Job drawing, mm, ordinate dimensions from the low corner. One solid piece. Give positions to 0.01 mm unless a question says otherwise; leave off trailing zeros. Order: outer loops, then holes, each group sorted by start corner. A loop starts at its lowest first (then second) coordinate and runs counter-clockwise, first axis right, second up.
Item 1: Band-saw the part on D-D on x = 29. Give the cut face in (y, z).
Item 2: Flat gauge pins, fed straight in: P1, Ø4, axis at x = 25.14, z = 22, coming from the +Y side; P2, Ø2.5, axis at x = 53.5, y = 2.5, coming from the +Z side (1 decimal). Where does each tip first touch, or does it go through?
Item 3: Band-saw the part on C-C on z = 35.5. Give the cut face in (x, y).
Item 4: Band-saw the part on A-A on z = 10.5. Give the cut face in (x, y) (1 decimal).
Item 5: Wall check: L1, parallel to Y at x = 32, z = 16; L2, parallel to Z at x = 30, y = 3; L3, parallel to X at y = 4.5, z = 20.5 (1 decimal). Give the ranges that are in metal, low to high.
Item 6: Band-saw the part on B-B on x = 51. Give the cut face in (y, z).
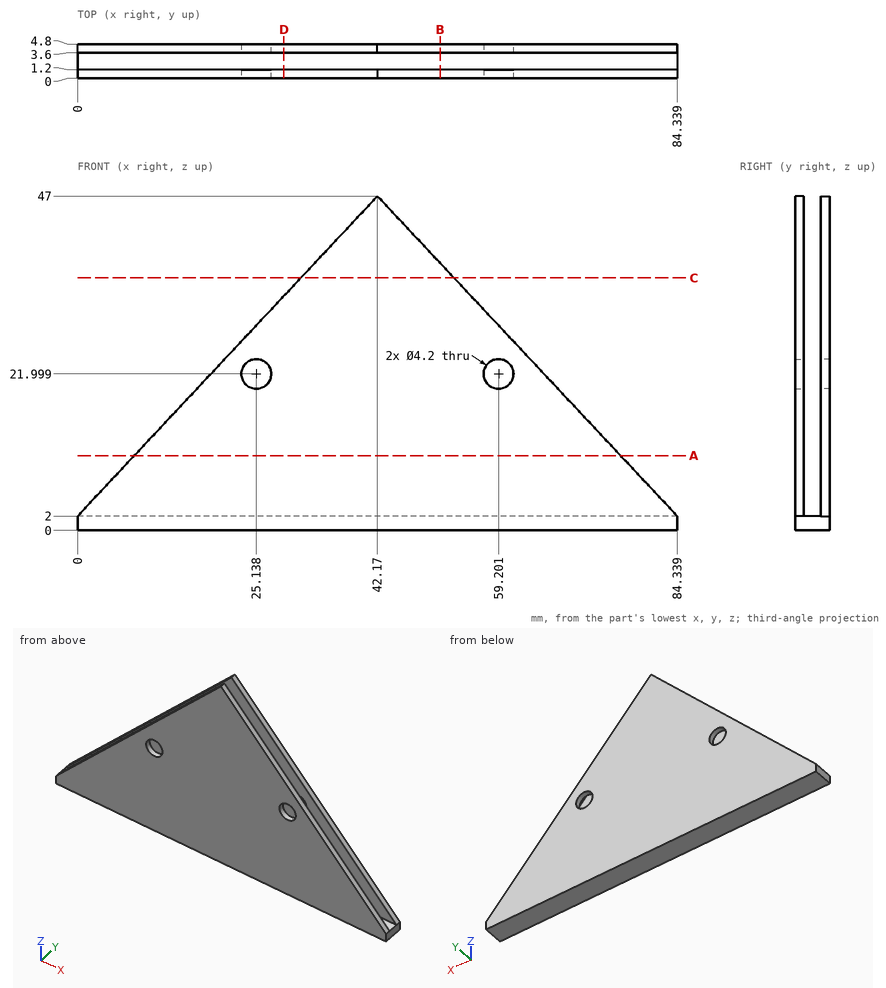
The answers:
1. outline: (0, 0) - (4.8, 0) - (4.8, 32.95) - (3.6, 32.95) - (3.6, 2) - (1.2, 2) - (1.2, 32.95) - (0, 32.95) - close
2. P1: passes through
2. P2: stops at z = 35.5
3. outline: (31.39, 0) - (52.95, 0) - (52.95, 1.2) - (31.39, 1.2) - close; (31.39, 3.6) - (52.95, 3.6) - (52.95, 4.8) - (31.39, 4.8) - close
4. outline: (8, 0) - (76.4, 0) - (76.4, 1.2) - (8, 1.2) - close; (8, 3.6) - (76.4, 3.6) - (76.4, 4.8) - (8, 4.8) - close
5. L1: y = 0 to 1.2, 3.6 to 4.8
5. L2: z = 0 to 2
5. L3: x = 17.3 to 23.7, 26.6 to 57.7, 60.7 to 67
6. outline: (0, 0) - (4.8, 0) - (4.8, 37.58) - (3.6, 37.58) - (3.6, 2) - (1.2, 2) - (1.2, 37.58) - (0, 37.58) - close
